from build123d import *

# Parameters (mm, degrees)
SKETCH1_W           = 160
SKETCH1_H           = 8
BOSS_EXTRUDE1_DEPTH = 160
SKETCH2_W           = 12.5
SKETCH2_H           = 8
BOSS_EXTRUDE2_DEPTH = 30
SKETCH3_W           = 12.63
SKETCH3_H           = 8
BOSS_EXTRUDE3_DEPTH = 30
SKETCH4_W           = 12.63
SKETCH4_H           = 8
BOSS_EXTRUDE4_DEPTH = 30
SKETCH5_W           = 12.63
SKETCH5_H           = 8
BOSS_EXTRUDE5_DEPTH = 30
SKETCH6_W           = 19
SKETCH6_H           = 10.5
SKETCH6_W_2         = 20.818922979
CUT_EXTRUDE1_DEPTH  = 10
SKETCH8_R           = 1.5
CUT_EXTRUDE4_DEPTH  = 25
SKETCH9_R           = 1.5
CUT_EXTRUDE5_DEPTH  = 25
BOSS_EXTRUDE6_START = 10
SKETCH10_R          = 4
BOSS_EXTRUDE6_DEPTH = 85
SKETCH13_R          = 2.7
CUT_EXTRUDE6_DEPTH  = 85
SKETCH14_R          = 2.7
CUT_EXTRUDE7_DEPTH  = 85


with BuildPart() as part:
    # Sketch1 → Boss-Extrude1 (new body)
    with BuildSketch(Plane(origin=(0, 0, 0), x_dir=(0, 0, -1), z_dir=(1, 0, 0))):
        Rectangle(SKETCH1_W, SKETCH1_H)
    extrude(amount=BOSS_EXTRUDE1_DEPTH)

    # Sketch2 → Boss-Extrude2 (add)
    with BuildSketch(Plane.XY.offset(80)):
        with Locations((6.25, 0)):
            Rectangle(SKETCH2_W, SKETCH2_H)
    extrude(amount=BOSS_EXTRUDE2_DEPTH)

    # Sketch3 → Boss-Extrude3 (add)
    with BuildSketch(Plane.XY.offset(80)):
        with Locations((153.685, 0)):
            Rectangle(SKETCH3_W, SKETCH3_H)
    extrude(amount=BOSS_EXTRUDE3_DEPTH)

    # Sketch4 → Boss-Extrude4 (add)
    with BuildSketch(Plane(origin=(0, 0, -80), x_dir=(-1, 0, 0), z_dir=(0, 0, -1))):
        with Locations((-153.685, 0)):
            Rectangle(SKETCH4_W, SKETCH4_H)
    extrude(amount=BOSS_EXTRUDE4_DEPTH)

    # Sketch5 → Boss-Extrude5 (add)
    with BuildSketch(Plane(origin=(0, 0, -80), x_dir=(-1, 0, 0), z_dir=(0, 0, -1))):
        with Locations((-6.315, 0)):
            Rectangle(SKETCH5_W, SKETCH5_H)
    extrude(amount=BOSS_EXTRUDE5_DEPTH)

    # Sketch6 → Cut-Extrude1 (cut)
    with BuildSketch(Plane(origin=(0, 4, 0), x_dir=(1, 0, 0), z_dir=(0, 1, 0))):
        with Locations((33.96830463, 33.015847685)):
            Rectangle(SKETCH6_W, SKETCH6_H)
        with Locations((33.058843141, -27.73153178)):
            Rectangle(SKETCH6_W_2, SKETCH6_H)
    extrude(amount=-CUT_EXTRUDE1_DEPTH, mode=Mode.SUBTRACT)

    # Sketch8 → Cut-Extrude4 (cut, symmetric)
    with BuildSketch(Plane.XY.offset(-38.265847685)):
        with Locations((33.619205895, 0)):
            Circle(SKETCH8_R)
    extrude(amount=CUT_EXTRUDE4_DEPTH, both=True, mode=Mode.SUBTRACT)

    # Sketch9 → Cut-Extrude5 (cut, symmetric)
    with BuildSketch(Plane.XY.offset(22.48153178)):
        with Locations((33.446786586, 0)):
            Circle(SKETCH9_R)
    extrude(amount=CUT_EXTRUDE5_DEPTH, both=True, mode=Mode.SUBTRACT)

    # Sketch10 → Boss-Extrude6 (add)
    with BuildSketch(Plane(origin=(0, 0, 0), x_dir=(1, 0, 0), z_dir=(0, 1, 0)).offset(BOSS_EXTRUDE6_START)):
        with Locations(Location((142.895014093, -27.73153178, 0), (0, 0, 270))):
            Circle(SKETCH10_R)
        with Locations(Location((142.895014093, 33.015847685, 0), (0, 0, 270))):
            Circle(SKETCH10_R)
    extrude(amount=-BOSS_EXTRUDE6_DEPTH)

    # Sketch13 → Cut-Extrude6 (cut)
    with BuildSketch(Plane(origin=(0, 10, 0), x_dir=(1, 0, 0), z_dir=(0, 1, 0))):
        with Locations(Location((142.895014093, -27.73153178, 0), (0, 0, 270))):
            Circle(SKETCH13_R)
    extrude(amount=-CUT_EXTRUDE6_DEPTH, mode=Mode.SUBTRACT)

    # Sketch14 → Cut-Extrude7 (cut)
    with BuildSketch(Plane(origin=(0, 10, 0), x_dir=(1, 0, 0), z_dir=(0, 1, 0))):
        with Locations(Location((142.895014093, 33.015847685, 0), (0, 0, 270))):
            Circle(SKETCH14_R)
    extrude(amount=-CUT_EXTRUDE7_DEPTH, mode=Mode.SUBTRACT)


solid = part.part
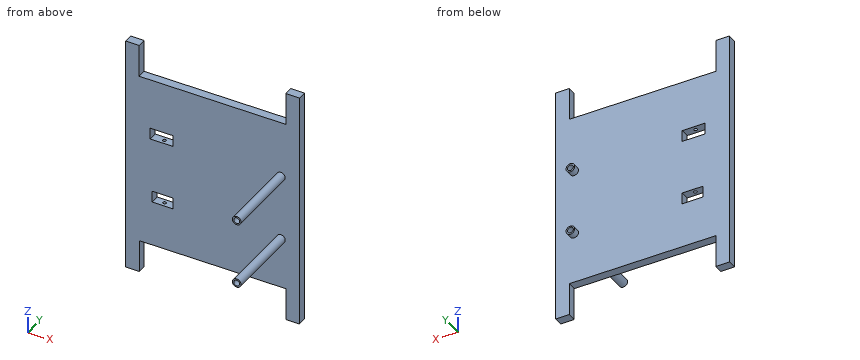
Model file for the job. Use its own axes, mm. Give positions to 0.01 mm unless a question says otherwise; leave off trailing zeros. Order: outer loops, then holes, each group sorted by start corner. A loop starts at its lowest first (then second) coordinate and runs counter-clockwise, first axis right, second up. Notation, with made-up numbers: (79.5, -6) -> (120.5, -6) arc R26 cw to (120.5, 23) -> close; hole circle Ø6 at (38.25, 42). An arc over 180 degrees is marked (long way). Use CSV: the item, a comma, the result in double quotes.
1. Band-saw the part on B-B, the plane x = 86. Give the cut face in (y, z).
Outcome:
outline,"(-4, -80) -> (4, -80) -> (4, 80) -> (-4, 80) -> close"
2. Band-saw the part on C-C, the plane y = -55.5. Give the cut face in (x, z), then the cut area to 3 significant figures.
Outcome:
outline,"circle Ø8 at (142.9, -33.02); circle Ø8 at (142.9, 27.73); hole circle Ø5.4 at (142.9, -33.02); hole circle Ø5.4 at (142.9, 27.73)"
area,"54.7 mm²"
3. Band-saw the part on A-A, the plane z = 11. Give the cut face in (x, y).
Outcome:
outline,"(0, -4) -> (160, -4) -> (160, 4) -> (0, 4) -> close; hole circle Ø3 at (33.45, 0)"
4. Drop flat-ended pins along their axis: pin 1 (4 mm diameter, centred on x = 33.45, y = 0, fed in from +Z); pin 2 (4 mm diameter, centred on x = 33.5, y = 0.5, fed in from -Z); pin 3 (3 mm diameter, centred on x = 85, z = 72, fed in from -Y). Give the stop position or say it passes through.
Outcome:
pin 1,"z = 80"
pin 2,"z = -80"
pin 3,"y = -4"
5. Drill centre lines: line 1 along X through (y, z) = (5.5, -32.5); line 2 along Y through (x, z) = (48.5, -57); line 3 along Z through (x, y) = (88.5, -3). Where is each one in solid material? Low to high. Write a range as from..to.
Outcome:
line 1,"138.93..140.24, 145.55..146.86"
line 2,"-4..4"
line 3,"-80..80"
